from build123d import *

# Parameters (mm, degrees)
BOSS_EXTRUDE1_DEPTH      = 2
BOSS_EXTRUDE1_DEPTH_BACK = 2
SKETCH2_R                = 1.5
FILLET1_R                = 3
FILLET2_R                = 1
CHAMFER1_SIZE            = 0.5


with BuildPart() as part:
    # Sketch2 → Boss-Extrude1 (new, two sides: drawn at the far end of the back side and taken through both)
    with BuildSketch(Plane(origin=(0, 0, 0), x_dir=(0, 0, -1), z_dir=(1, 0, 0)).offset(-BOSS_EXTRUDE1_DEPTH_BACK)):
        with BuildLine():
            ThreePointArc((4, 2.5), (6.5, 0), (4, -2.5))
            Line((4, -2.5), (2, -2.5))
            Line((2, -2.5), (2, -9.5))
            Line((2, -9.5), (-4, -9.5))
            Line((-4, -9.5), (-6, -7.5))
            Line((-6, -7.5), (-6, -6.5))
            Line((-6, -6.5), (-5, -6.5))
            Line((-5, -6.5), (-4, -7.5))
            Line((-4, -7.5), (0, -7.5))
            Line((0, -7.5), (0, 7.5))
            Line((0, 7.5), (-2, 7.5))
            Line((-2, 7.5), (-2, 9.5))
            Line((-2, 9.5), (2, 9.5))
            Line((2, 9.5), (2, 2.5))
            Line((2, 2.5), (4, 2.5))
        make_face()
        with Locations((4, 0)):
            Circle(SKETCH2_R, mode=Mode.SUBTRACT)
    extrude(amount=BOSS_EXTRUDE1_DEPTH + BOSS_EXTRUDE1_DEPTH_BACK)

    # Fillet1
    fillet1_edges = [part.edges().sort_by_distance(p)[0] for p in [
        (0, 2.5, -2),
        (0, -2.5, -2),
    ]]
    fillet(fillet1_edges, radius=FILLET1_R)

    # Fillet2
    fillet2_edges = [part.edges().sort_by_distance(p)[0] for p in [
        (0, -9.5, -2),
        (0, -9.5, 4),
        (0, -7.5, 6),
        (0, 9.5, 2),
        (0, 9.5, -2),
    ]]
    fillet(fillet2_edges, radius=FILLET2_R)

    # Chamfer1
    chamfer1_edges = [part.edges().sort_by_distance(p)[0] for p in [
        (2, -8.5, 5),
        (2, -9.5, 1.292893219),
        (2, -6.954163457, -2),
        (2, 9.207106781, -1.707106781),
        (2, -9.207106781, -1.707106781),
        (2, -9.423879533, 3.96846987),
        (2, -7.46846987, 5.923879533),
        (2, 9.207106781, 1.707106781),
        (-2, 8, 2),
        (-2, -6.954163457, -2),
        (-2, -9.5, 1.292893219),
        (-2, -8.5, 5),
        (-2, 9.207106781, -1.707106781),
        (-2, -9.207106781, -1.707106781),
        (-2, -9.423879533, 3.96846987),
        (-2, -7.46846987, 5.923879533),
        (-2, 9.207106781, 1.707106781),
        (-2, 7.5, 1),
        (-2, 0, 0),
        (-2, -7.5, 2),
        (2, 0, -2.5),
        (2, 7.5, 1),
        (-2, -7, 4.5),
        (2, 0, 0),
        (2, -7.5, 2),
        (2, -7, 4.5),
        (2, -6.5, 5.5),
        (2, -6.792893219, 6),
        (-2, -6.5, 5.5),
        (-2, -6.792893219, 6),
        (-2, 0, -2.5),
        (2, 0, -6.5),
        (-2, 0, -6.5),
        (2, 6.954163457, -2),
        (-2, 6.954163457, -2),
        (2, 3.489495707, -2.693902257),
        (-2, 3.489545225, -2.693861055),
        (2, -3.489545225, -2.693861055),
        (-2, -3.489545225, -2.693861055),
        (2, 9.5, 0),
        (-2, 9.5, 0),
        (2, 8, 2),
    ]]
    chamfer(chamfer1_edges, length=CHAMFER1_SIZE - 0.0001)  # a hair under: the kernel refuses the full size


solid = part.part
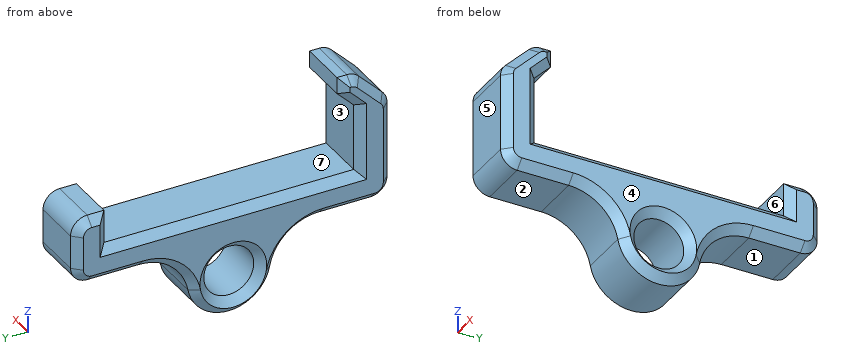
Could you check a few things on this model? Use its own coordinates, in mm. Face numbers are marked on the shaded views. A direction names the side the tool comes from. Give positions to 0.01 mm unless a question says otherwise; leave off trailing zeros. Write each loop counter-clockwise with the first axis right and the second up, starting at its lowest first coordinate (ties: lowest second). Pieces come first, ordered by that corner, then holes. Notation, with made-up numbers: (44.5, 58.25) -> (63.5, 58.25) arc R22 cw to (63.5, 72.25) -> close; hole circle Ø4 at (-17.75, -21). An arc over 180 degrees is marked (long way). Answer as CSV lines item,"result". Start each with the question number.
(1) Which directions (+Z, -Z, +X, -X, +Y, -Y) give clear straight access to the entire face, cutting with the end or side of a thin tool? Please do the marked faces 1, 2 and 3.
(2) If we section it at B-B, the plane y = 6: Write out the boundary of the cut face in (x, z).
(3) If we mould it in two halves opening along Y, with no side actions, what happens to the marked faces 4, 5, 6 and 7? For each: +Y half, -Y half, draft (parallel to the pull), parting line (faces both ways), or undercut.
(4) I'm going to push flat-ended pins straight in: pin 1 Ø5 at (y, z) = (0, -4) entering from -X; pin 2 Ø1.5 at (x, y) = (1, -4.5) entering from +Z; pin 3 Ø0.8 at (x, z) = (-0.5, 5.5) entering from +Y; pin 4 Ø1 at (x, y) = (-0.5, -1.5) entering from -Z. Where does each tip first touch, or does it pass through?
(5) Please list where these lines run through material, in increasing order: line 1 (Y direction, x = 1.2, z = -3.5); line 2 (Z direction, x = 1.15, y = 0.5); line 3 (Y direction, x = -0.2, z = 2.5).
Answer list:
1,face 1,"-Z, +X, -X, +Y"
1,face 2,"-Z, +X, -X, -Y"
1,face 3,"+X, -X"
2,outline,"(-2, -1.5) -> (-1.5, -2) -> (1.5, -2) -> (2, -1.5) -> (2, -0.5) -> (1.5, 0) -> (-1.5, 0) -> (-2, -0.5) -> close"
3,face 4,"draft"
3,face 5,"-Y half"
3,face 6,"undercut"
3,face 7,"undercut"
4,pin 1,"x = -2"
4,pin 2,"z = 0"
4,pin 3,"y = -6.5"
4,pin 4,"z = -6.29"
5,line 1,"-2.81 to -1.41, 1.41 to 2.81"
5,line 2,"-6.45 to -5.41, -2.59 to 0"
5,line 3,"-9.5 to -7.5"
